```python
from build123d import *

# Parameters (mm, degrees)
F0_R      = 52
F1_DEPTH  = 75
F2_R      = 7
F3_DEPTH  = 2
F1_FACE_R = 52
F3_FACE_R = 7
F7_T      = -2
F8_R      = 5
F9_DEPTH  = 25
F10_R     = 62
F10_R_2   = 52
F11_DEPTH = 5
F13_D     = 3
F15_R     = 1.25
F17_R     = 5


with BuildPart() as f1:
    # F0 (on Top) → F1 (new body)
    with BuildSketch(Plane.XY):
        Circle(F0_R)
    extrude(amount=F1_DEPTH)


with BuildPart() as f3:
    # F2 (on face) → F3 (new body)
    with BuildSketch(Plane.XY.offset(75)):
        Circle(F2_R)
    extrude(amount=F3_DEPTH)


with BuildPart() as f3_1:
    # F4: moved
    add(f3.part.moved(Location((0, 0, 50))))


with BuildPart() as f5:
    # F1_face (on face) → F5 section 0
    with BuildSketch(Plane.XY.offset(75)):
        Circle(F1_FACE_R)
    # F3_face (on face) → F5 section 1
    with BuildSketch(Plane(origin=(0, 0, 125), x_dir=(1, 0, 0), z_dir=(0, 0, -1))):
        Circle(F3_FACE_R)
    loft()

    # F6: union F3, F1
    add(f3_1.part)
    add(f1.part)

    # F7
    f7_openings = [f5.faces().sort_by_distance(p)[0] for p in [
        (0, 0, 0),
    ]]
    offset(amount=F7_T, openings=f7_openings, kind=Kind.INTERSECTION)

    # F8 (on face) → F9 (cut)
    with BuildSketch(Plane.XY.offset(127)):
        Circle(F8_R)
    extrude(amount=-F9_DEPTH, mode=Mode.SUBTRACT)

    # F10 (on face) → F11 (join)
    with BuildSketch(Plane(origin=(0, 0, 0), x_dir=(1, 0, 0), z_dir=(0, 0, -1))):
        Circle(F10_R)
        Circle(F10_R_2, mode=Mode.SUBTRACT)
    extrude(amount=-F11_DEPTH)

    # F13 (through all)
    with Locations(Plane.XY.offset(5)):
        with Locations((0, 57), (40.3050865276, 40.3050865276), (57, 0), (40.3050865276, -40.3050865276), (0, -57), (-40.3050865276, -40.3050865276), (-57, 0), (-40.3050865276, 40.3050865276)):
            Hole(F13_D / 2)

    # F16: sweep along a path in F14
    with BuildLine(Plane(origin=(0, 0, 0), x_dir=(1, 0, 0), z_dir=(0, 0, -1))) as f16_path:
        CenterArc((0, 0), 52.5, 0, 360)
    # F15 (on Front) → F16 (sweep, cut)
    with BuildSketch(Plane.XZ):
        with Locations((-52.4801053107, 0)):
            Circle(F15_R)
    sweep(path=f16_path.line, mode=Mode.SUBTRACT)

    # F17
    f17_edges = [f5.edges().sort_by_distance(p)[0] for p in [
        (-52, 0, 75),
    ]]
    fillet(f17_edges, radius=F17_R)


solid = f5.part
```
Here's how the part is built. I have some questions about the finished solid (model axes, mm). A direction names the side the tool comes from. Coordinates: 2 decimals unless noted, no trailing zeros. Loops run counter-clockwise (first coordinate to the right, second up) from the corner with the lowest first, then second, coordinate; pieces in that order, holes last. Notation, with made-up numbers: (22.25, -10) - (72.25, -10) arc R30 cw to (72.25, 17) - close; hole circle Ø10 at (-9.75, 16). An arc over 180 degrees is marked (long way). Return JSON: item names as keys, results as strings. Group by question number.
Item 1: If we section it at A-A on z = 11.5: Write out the boundary of the cut face in (x, y), and give its area (3 significant figures).
Item 2: On a 3-axis mill with a long thin cutter (end or side, diameter ignored), from which of +Z, -Z, +X, -X, +Y, -Y can I reach the whole of each face in a straight line? I mean faces 4 (the face through (47.69, 15.02, 36.6)), 5 (the face through (-8.071, -61.472, 2.465)), 6 (the face through (-41.265, -31.641, 38.564)). Say none if no direction works.
Item 3: I need wall thicknesses on line 1 (Y direction, x = 0, z = 1.1); line 2 (Y direction, x = 0, z = 31); line 3 (Y direction, x = -18, z = 21). Which ranges of each line are inside material? Lowest first, please. Write a range as from..to.
Item 4: Will these pins go through, and if not, where does the flat tip stop? P1, Ø6, axis at y = 2.5, z = 92, coming from the -X side; P2, Ø12, axis at x = -45.5, z = 65.5, coming from the +Y side; P3, Ø4, axis at x = 40.5, y = -21.5, coming from the -Z side.
Item 5: If we section it at B-B on z = 79.5: Write out the boundary of the cut face in (x, y).
Item 6: We'd pull the mould along Y, two halves only. Please class faces 1 (the face through (-32, -42, 5)), 2 (the face through (-1.08, -4.88, 125.6)), 3 (the face through (6.466, -2.681, 125.986)): +Y half, -Y half, draft (parallel to the pull), parting line (faces both ways), or undercut.
Calculated:
{
 "1": {"outline": "circle Ø104 at (0, 0); hole circle Ø100 at (0, 0)", "area": "641 mm^2"},
 "2": {"face 4": "-Z", "face 5": "+Z, -Z", "face 6": "+Z"},
 "3": {"line 1": "y = -62..-58.5, -55.5..-53.07, -51.89..-50, 50..51.89, 53.07..55.5, 58.5..62", "line 2": "y = -52..-50, 50..52", "line 3": "y = -48.79..-46.65, 46.65..48.79"},
 "4": {"P1": "stops at x = -39.33", "P2": "stops at y = 33.82", "P3": "stops at z = 76.62"},
 "5": {"outline": "circle Ø95.9 at (0, 0); hole circle Ø90.52 at (0, 0)"},
 "6": {"face 1": "draft", "face 2": "undercut", "face 3": "parting line"}
}
